Geometry: see drawing. Coordinates: mm, zero at the bounding-box minimum. A direction names the side the tool comes from. Coordinates: 2 decimals unless noted, no trailing zeros. Write each loop counter-clockwise with the first axis right and the second up, starting at its lowest first coordinate (ties: lowest second). Pieces come first, ordered by that corner, then holes. Notation, with made-up numbers: (58, -37) - (103, -37) arc R14 cw to (103, -28) - close; hole circle Ø6 at (5.5, 70). An arc over 180 degrees is marked (long way). Use a Markdown table: item, result. Add a question column.
Q1. Material intervals for probe 1 along X at (y, z) = (22.5, 4.25) (1 decimal); probe 2 along Z at (x, y) = (12, 18.75) (1 decimal); probe 3 along X at (y, z) = (4, 3) (1 decimal), sorted ascending. Write a range as from..to.
Q2. Mould query, pull axis Z, two halves, no side actions, for the marked faces 3, 4 and 5. Classes: released by +Z, released by -Z, zero draft, split by the parting line, or undercut.
Q3. Set-up query: the marked faces 1 and 2. Return all of +Z, -Z, +X, -X, +Y, -Y with unobstructed straight access to the full face (end or side cutting, diameter ignored); none if empty.
Q4. Pin query (flat end, axial travel): P1, Ø7.5, axis at x = 9.5, z = 9.5, coming from the -Y side; P2, Ø1, axis at x = 6.5, y = 15, coming from the +Z side; P3, Ø1.6, axis at x = 2.5, y = 9, coming from the +Z side (1 decimal); P4, Ø1, axis at y = 9, z = 12, coming from the +X side (1 decimal). Return the tip coordinate at first contact, or that it passes through.
Q5. Section query A-A (x = 7.5). Return the cut outline in (y, z).
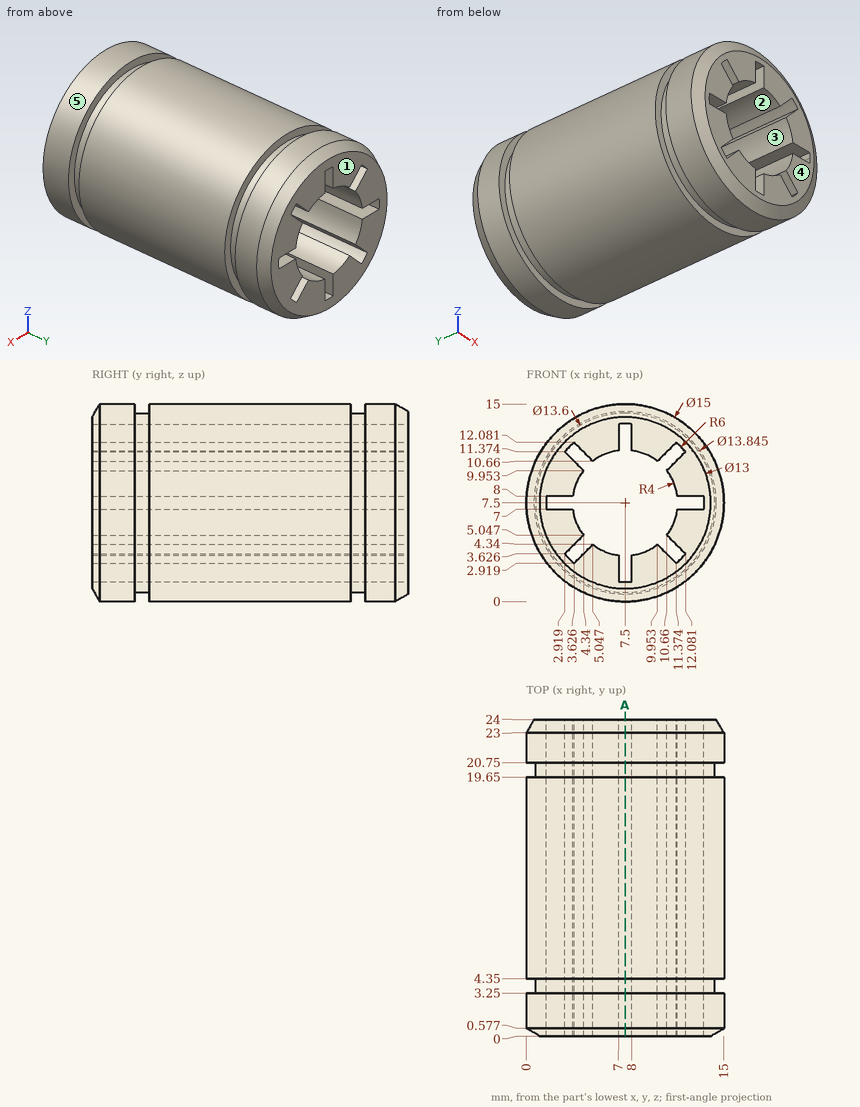
Values follow:
| question | item | result |
|---|---|---|
| 1 | probe 1 | 0.7..3.5, 5..5.2, 9.8..10, 11.5..14.3 |
| 1 | probe 2 | 1.5..3.5, 3.7..7, 8..11.3, 11.5..13.5 |
| 1 | probe 3 | 2.4..3.5, 3.7..7, 8..11.3, 11.5..12.6 |
| 2 | face 3 | undercut |
| 2 | face 4 | zero draft |
| 2 | face 5 | split by the parting line |
| 3 | face 1 | +Z, -Z, +X, -X, +Y |
| 3 | face 2 | +Y, -Y |
| 4 | P1 | y = 0 |
| 4 | P2 | z = 14.98 |
| 4 | P3 | z = 13.7 |
| 4 | P4 | x = 13.8 |
| 5 | outline | (0, 1) - (0.58, 0) - (3.25, 0) - (3.25, 0.7) - (4.35, 0.7) - (4.35, 0) - (19.65, 0) - (19.65, 0.7) - (20.75, 0.7) - (20.75, 0) - (23, 0) - (24, 0.58) - (24, 1.5) - (0, 1.5) - close; (0, 13.5) - (24, 13.5) - (24, 14.42) - (23, 15) - (20.75, 15) - (20.75, 14.3) - (19.65, 14.3) - (19.65, 15) - (4.35, 15) - (4.35, 14.3) - (3.25, 14.3) - (3.25, 15) - (0.58, 15) - (0, 14) - close |
